Source: CAD feature listing. Evaluate the final solid. Frame: model axes, mm. A direction names the side the tool comes from. Give positions to 0.01 mm unless a question says otherwise; leave off trailing zeros. Order: outer loops, then holes, each group sorted by start corner. A loop starts at its lowest first (then second) coordinate and runs counter-clockwise, first axis right, second up.
1) Draft query along Z for faces 4 (the face through (-6.3, 28.7, 0.8)), 5 (the face through (-1, 12.7, 0)), 6 (the face through (4.2, 35, 0)), 7 (the face through (7.21, 7.53, -0.15)). Return one class per face: released by +Z, released by -Z, zero draft, split by the parting line, or undercut.
2) Section A-A, the plane y = 4. Return loops of the section in (x, z) (3 decimals), plus the area to 3 significant figures.
3) Access query for faces 1 (the face through (-5.796, 6.54, -7.559)), 2 (the face through (5, 31.75, 0)), 3 (the face through (4.957, 8, 0)). Directions: +Z, -Z, +X, -X, +Y, -Y. A direction counts if a zero-diameter tool reaches every point of the face in a straight line with its end or side. Return the directions, or none.
4) Material intervals for line 1 (Y direction, x = 3.5, z = -0.75); line 2 (Z direction, x = 0.25, y = 31); line 3 (X direction, y = 10.5, z = 2.5), sorted ascending.
5) First-contact query: P1, Ø5.5, axis at x = -3.5, z = 2.5, coming from the -Y side; P2, Ø4, axis at x = 0, y = 27.5, coming from the +Z side; P3, Ø4, axis at y = 15, z = 6, coming from the +X side; P4, Ø1, axis at x = -7.5, z = 6, coming from the +Y side. Flat tips, straight axial feed; report the tip coordinate or a pass-through.
6) Section B-B, the plane y = 36. Return loops of the section in (x, z).
```python
from build123d import *

# Parameters (mm, degrees)
SKETCH1_R           = 9.525
MALE_END_DEPTH      = 15.875
SKETCH2_R           = 6.35
FEMALE_END_DEPTH    = 38.1
UPPER_R             = 4.7625
LOWER_R             = 4.7625
D_CUT_DEPTH         = 12.7
SET_HOLE_REACH      = 43.858
SET_HOLE_END_RADIUS = 9.525
SKETCH5_R           = 1.190625
D_START             = -6.35
D_BOSS_DEPTH        = 6.35
EDGE_CHAMFER_SIZE   = 0.79375


with BuildPart() as part:
    # Sketch1 → male end (new body)
    with BuildSketch(Plane(origin=(0, 0, 0), x_dir=(1, 0, 0), z_dir=(0, 1, 0))):
        with Locations(Location((0, 0, 0), (0, 0, 270))):
            Circle(SKETCH1_R)
    extrude(amount=MALE_END_DEPTH)

    # Sketch2 → female end (add)
    with BuildSketch(Plane(origin=(0, 0, 0), x_dir=(-1, 0, 0), z_dir=(0, 1, 0))):
        with Locations(Location((0, 0, 0), (0, 0, 270))):
            Circle(SKETCH2_R)
    extrude(amount=FEMALE_END_DEPTH)

    # upper
    # the kernel refuses this fillet: 4.7625 mm, written as the material it adds along each edge
    with BuildSketch(Plane(origin=(0, 15.875, 0), x_dir=(0, 0, -1), z_dir=(-1, 0, 0))) as upper_piece_1:
        with BuildLine():
            CenterArc((11.1125, -4.490128061), UPPER_R, 109.471220634, 70.528779366)
            Line((6.35, -4.490128061), (6.25475, -4.490128061))
            Line((6.25475, -4.490128061), (6.25475, 0))
            Line((6.25475, 0), (6.35, 0.09525))
            ThreePointArc((6.35, 0.09525), (7.9375, 0.09525), (9.49325, 0.089802561))
            Line((9.49325, 0.089802561), (9.525, 0))
        make_face()
    revolve(axis=Axis((0, 15.875, 0), (0, -1, 0)))

    # lower
    lower_edges = [part.edges().sort_by_distance(p)[0] for p in [
        (9.525, 15.875, 0),
    ]]
    fillet(lower_edges, radius=LOWER_R)

    # Sketch3 → D cut (cut)
    with BuildSketch(Plane.XZ):
        with BuildLine():
            Line((4.956967161, -3.96875), (4.956967161, 3.96875))
            ThreePointArc((4.956967161, 3.96875), (-6.35, 0), (4.956967161, -3.96875))
        make_face()
    extrude(amount=-D_CUT_DEPTH, mode=Mode.SUBTRACT)

    # set hole: up to this cylinder (the profile starts inside it)
    set_hole_end = Plane(origin=(0, 6.35, 0), z_dir=(0, -1, 0)) * Cylinder(SET_HOLE_END_RADIUS, 107.766, mode=Mode.PRIVATE)
    # Sketch5 → set hole (cut, up to the surface)
    with BuildSketch(Plane.ZY.offset(-4.956967161), mode=Mode.PRIVATE) as set_hole_sk1:
        with Locations((0, 6.35)):
            Circle(SKETCH5_R)
    set_hole_tool1 = extrude(set_hole_sk1.sketch, amount=-SET_HOLE_REACH, mode=Mode.PRIVATE) & set_hole_end
    add(set_hole_tool1.solids().sort_by_distance((4.956967, 6.35, 0))[0], mode=Mode.SUBTRACT)

    # Sketch4 → D boss (cut)
    with BuildSketch(Plane(origin=(0, 38.1, 0), x_dir=(-1, 0, 0), z_dir=(0, 1, 0)).offset(D_START)):
        with BuildLine():
            Line((-4.200130206, 4.7625), (-4.200130206, -4.7625))
            ThreePointArc((-4.200130206, -4.7625), (-6.35, 0), (-4.200130206, 4.7625))
        make_face()
    extrude(amount=D_BOSS_DEPTH, mode=Mode.SUBTRACT)

    # edge chamfer
    edge_chamfer_edges = [part.edges().sort_by_distance(p)[0] for p in [
        (-5.939881102, 38.1, 2.24506403),
    ]]
    chamfer(edge_chamfer_edges, length=EDGE_CHAMFER_SIZE)


solid = part.part
```
From the geometry:
1. face 4: split by the parting line
1. face 5: undercut
1. face 6: zero draft
1. face 7: undercut
2. outline: circle Ø19.05 at (0, 0); hole (4.957, -3.969) - (4.957, 3.969) arc R6.35 ccw (long way) to start
2. area: 166 mm2
3. face 1: +Y, -Y
3. face 2: +Z, -Z, +X, +Y
3. face 3: -Y
4. line 1: y = 12.7 to 38.1
4. line 2: z = -6.35 to 6.35
4. line 3: x = -9.19 to -5.84, 4.96 to 9.19
5. P1: stops at y = 0
5. P2: stops at z = 6.35
5. P3: stops at x = 8.46
5. P4: stops at y = 15.22
6. outline: (4.2, -4.76) - (4.2, 4.76) arc R6.35 ccw (long way) to start
